Geometry check sheet. Reference: the model listing, model coordinates, mm. A direction names the side the tool comes from. Round coordinates to 2 decimals unless told otherwise and drop trailing zeros. Order: outer loops, then holes, each group sorted by start corner. A loop starts at its lowest first (then second) coordinate and runs counter-clockwise, first axis right, second up. Notation, with made-up numbers: M 50,10.5 L 98,10.5 A22 ccw 98,40.5 Z; hole C -28,32.5 d7. An arc over 180 degrees is marked long. Return JSON: item names as keys, results as strings. Group by question number.
```python
from build123d import *

# Parameters (mm, degrees)
F1_DEPTH       = 15
F2_D           = 9
F3_D           = 6.6
F4_R           = 9.99999
F5_D           = 25
F5_CBORE_D     = 28
F5_CBORE_DEPTH = 12
F6_D           = 5.5
F6_CBORE_D     = 9.75
F6_CBORE_DEPTH = 5
F7_W           = 40
F7_H           = 80
F8_DEPTH       = 5


# Not quite as in the source:
# - a fillet or chamfer is up to 0.001 mm smaller than in the source, because OpenCascade refuses the exact size


with BuildPart() as f1:
    # F0 (on Front) → F1 (new body)
    with BuildSketch(Plane.XZ):
        Polygon((62.0740194619, 20.9148037434), (-57.9259805381, 20.9148037434), (-62.9259805381, 20.9148037434), (-62.9259805381, -39.0851962566), (-57.9259805381, -39.0851962566), (-7.9259805381, -39.0851962566), (-7.9259805381, -119.0851962566), (162.0740194619, -119.0851962566), (162.0740194619, -99.0851962566), (62.0740194619, -99.0851962566), align=None)
    extrude(amount=F1_DEPTH)

    # F2 (through all)
    with Locations(Plane(origin=(0, 0, 0), x_dir=(1, 0, 0), z_dir=(0, 1, 0))):
        with Locations((24.0740194619, 79.0851962566), (24.0740194619, 39.0851962566)):
            Hole(F2_D / 2)

    # F3 (through all)
    with Locations(Plane(origin=(0, 0, 0), x_dir=(1, 0, 0), z_dir=(0, 1, 0))):
        with Locations((24.0740194619, 109.0851962566), (74.0740194619, 109.0851962566), (124.0740194619, 109.0851962566)):
            Hole(F3_D / 2)

    # F4 (radius 10 in the source; OpenCascade refuses exactly that, so slightly less here)
    f4_edges = [f1.edges().sort_by_distance(p)[0] for p in [
        (62.074019, -7.5, 20.914804),
        (62.074019, -7.5, -99.085196),
        (162.074019, -7.5, -119.085196),
        (162.074019, -7.5, -99.085196),
        (-7.925981, -7.5, -119.085196),
        (-7.925981, -7.5, -39.085196),
        (-62.925981, -7.5, 20.914804),
        (-62.925981, -7.5, -39.085196),
    ]]
    fillet(f4_edges, radius=F4_R)

    # F5 (through all)
    with Locations(Plane(origin=(0, 0, 0), x_dir=(1, 0, 0), z_dir=(0, 1, 0))):
        with Locations((-29.9259805381, 9.0851962566)):
            CounterBoreHole(F5_D / 2, F5_CBORE_D / 2, F5_CBORE_DEPTH)

    # F6 (through all)
    with Locations(Plane(origin=(0, 0, 0), x_dir=(1, 0, 0), z_dir=(0, 1, 0))):
        with Locations((-53.4959805381, -14.4848037434), (-6.3559805381, -14.4848037434), (-6.3559805381, 32.6551962566), (-53.4959805381, 32.6551962566)):
            CounterBoreHole(F6_D / 2, F6_CBORE_D / 2, F6_CBORE_DEPTH)

    # F7 (on face) → F8 (cut)
    with BuildSketch(Plane.XZ):
        with Locations((24.0740194619, -59.0851962566)):
            Rectangle(F7_W, F7_H)
    extrude(amount=F8_DEPTH, mode=Mode.SUBTRACT)


solid = f1.part
```
Q1. Section check A-A on x = -34.5. Record the cut outline in (y, z).
Q2. Set-up check for faces 4 (the face through (-7.926, -7, -79)), 5 (the face through (113, -7, -99.085)), 6 (the face through (-59.92, -7.6, 18.06)), 7 (the face through (-50.88, -2.46, -36.77)): record each of +Z, -Z, +X, -X, +Y, -Y from which the full face is reachable in a straight line by a thin tool's end or side.
Q3. Release check for a two-part mould opening along Z. For faces 1 (the face through (49, 0, -49)), 2 (the face through (-36.646, -13.521, -19.625)), 3 (the face through (59.07, -7.6, 18.06)) record: +Z half, -Z half, draft (parallel to the pull), parting line (faces both ways), or undercut.
Q4. Section check B-B on x = 14.5. Record the cut outline in (y, z), plus the area to 3 significant figures.
Q5. Section check D-D on x = 118. Record the cut outline in (y, z).
Q6. Depth check by flat-ended pin: pin 1 Ø5.5 at (y, z) = (-2, -45.5) entering from +X; pin 2 Ø9 at (x, z) = (-53.5, 14.48) entering from +Y; pin 3 Ø4.5 at (y, z) = (-7, -82.5) entering from -X; pin 4 Ø8 at (x, z) = (24.07, -39.09) entering from -Y. Enter the tip coordinate at first touch or a pass-through.
Q7. Section check C-C on y = -8.75. Count the separate pieces of the cut face and the enclosed holes in it, plus the area to 3 significant figures.
Q8. Material ranges on line 1 along X through (y, z) = (-3, -82); line 2 along Z through (x, y) = (19, -1.75); line 3 along X through (y, z) = (-3.5, 10), recorded low to high.
Geometry check:
{
 "1": {"outline": "M -15,-39.09 L 0,-39.09 L 0,-22.32 L -12,-22.32 L -12,-20.72 L -15,-20.72 Z; M -15,2.55 L -12,2.55 L -12,4.15 L 0,4.15 L 0,20.91 L -15,20.91 Z"},
 "2": {"face 4": "-Z, -X, +Y, -Y", "face 5": "+Z, +X, +Y, -Y", "face 6": "+Z, -X, +Y, -Y", "face 7": "+Y"},
 "3": {"face 1": "draft", "face 2": "undercut", "face 3": "+Z half"},
 "4": {"outline": "M -15,-119.09 L 0,-119.09 L 0,-99.09 L -5,-99.09 L -5,-19.09 L 0,-19.09 L 0,20.91 L -15,20.91 Z", "area": "1,700 mm^2"},
 "5": {"outline": "M -15,-119.09 L 0,-119.09 L 0,-99.09 L -15,-99.09 Z"},
 "6": {"pin 1": "stops at x = 62.07", "pin 2": "stops at y = -5", "pin 3": "stops at x = -7.93", "pin 4": "passes through"},
 "7": {"separate pieces": "1", "enclosed holes": "10", "area": "14,100 mm^2"},
 "8": {"line 1": "x = -7.93 to 4.07, 44.07 to 62.07", "line 2": "z = -119.09 to -99.09, -19.09 to 20.91", "line 3": "x = -62.93 to -55.41, -51.58 to -8.27, -4.44 to 62.07"}
}
